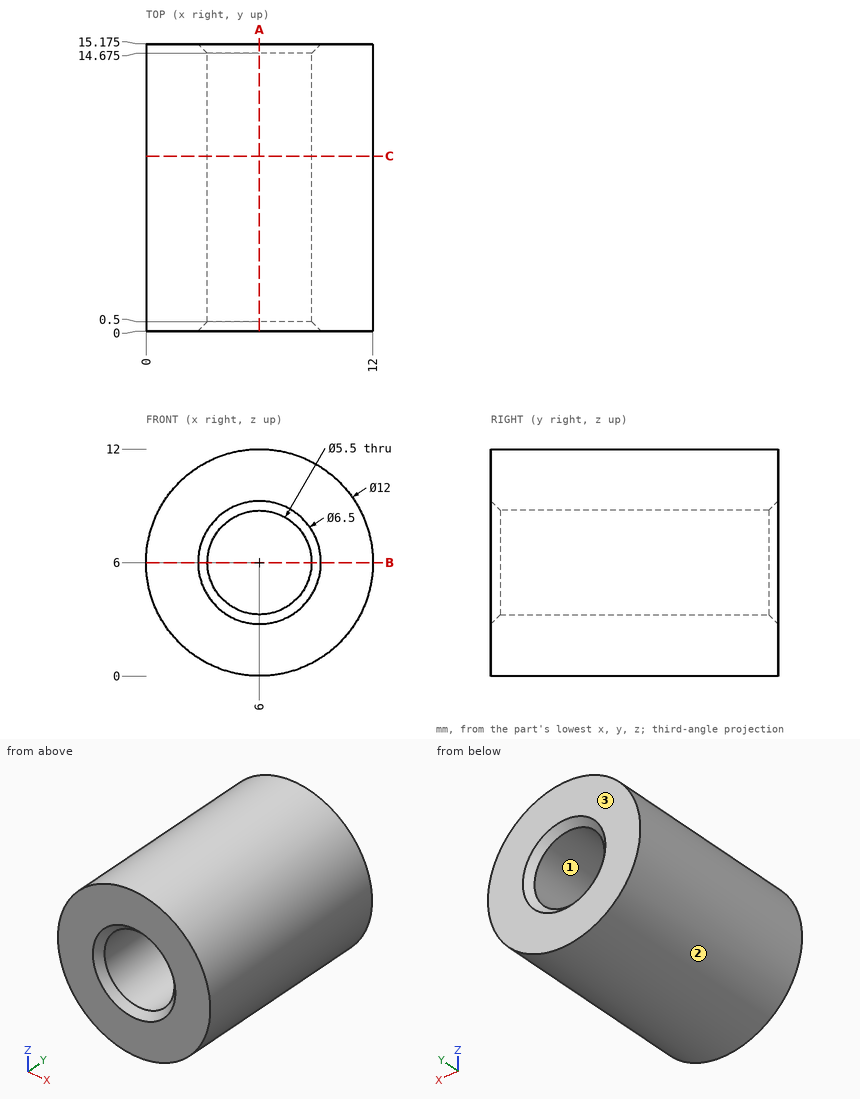
Input: dimensioned drawing with shaded views. Units: mm. Origin: part minimum x, y, z. Give positions to 0.01 mm unless a question says otherwise; leave off trailing zeros. Order: outer loops, then holes, each group sorted by start corner. A loop starts at its lowest first (then second) coordinate and runs counter-clockwise, first axis right, second up. Notation, with made-up numbers: (46.25, 31) -> (104.25, 31) arc R21 cw to (104.25, 38) -> close; hole circle Ø2 at (73, 87.25). An arc over 180 degrees is marked (long way). Use a Markdown table: item, result.
1) Section query A-A, the plane x = 6. Return the cut outline in (y, z) (3 decimals), then the cut area to 3 significant figures.
Answer list:
| item | result |
|---|---|
| outline | (0, 0) -> (15.175, 0) -> (15.175, 2.75) -> (14.675, 3.25) -> (0.5, 3.25) -> (0, 2.75) -> close; (0, 9.25) -> (0.5, 8.75) -> (14.675, 8.75) -> (15.175, 9.25) -> (15.175, 12) -> (0, 12) -> close |
| area | 98.1 mm² |
2) Section query C-C, the plane y = 9.25. Return the cut outline in (x, z), then the cut area to 3 significant figures.
Answer list:
| item | result |
|---|---|
| outline | circle Ø12 at (6, 6); hole circle Ø5.5 at (6, 6) |
| area | 89.3 mm² |
3) Ray query, line 1 along X through (y, z) = (5.75, 6); line 2 along Z through (x, y) = (6.25, 12.75); line 3 along Z through (x, y) = (6.75, 7.75). Return the intervals inside material, ascending. Write a range as [from, to].
Answer list:
| item | result |
|---|---|
| line 1 | [0, 3.25], [8.75, 12] |
| line 2 | [0.01, 3.26], [8.74, 11.99] |
| line 3 | [0.05, 3.35], [8.65, 11.95] |
4) Mould query, pull axis Z, two halves, no side actions, for the marked faces 1, 2 and 3. Classes: +Z half, -Z half, draft (parallel to the pull), parting line (faces both ways), or undercut.
Answer list:
| item | result |
|---|---|
| face 1 | undercut |
| face 2 | parting line |
| face 3 | draft |
5) Contact query for flat-ended pins moving along their axis: P1, Ø6, axis at y = 7.5, z = 11, coming from the +X side; P2, Ø5, axis at x = 6, z = 6, coming from the +Y side; P3, Ø3, axis at y = 9.5, z = 10.5, coming from the +X side. Output: stop coordinate, or through.
Answer list:
| item | result |
|---|---|
| P1 | x = 11.66 |
| P2 | through |
| P3 | x = 11.2 |
6) Section query B-B, the plane z = 6. Return the cut outline in (x, y) (3 decimals).
Answer list:
| item | result |
|---|---|
| outline | (0, 0) -> (2.75, 0) -> (3.25, 0.5) -> (3.25, 14.675) -> (2.75, 15.175) -> (0, 15.175) -> close; (8.75, 0.5) -> (9.25, 0) -> (12, 0) -> (12, 15.175) -> (9.25, 15.175) -> (8.75, 14.675) -> close |
